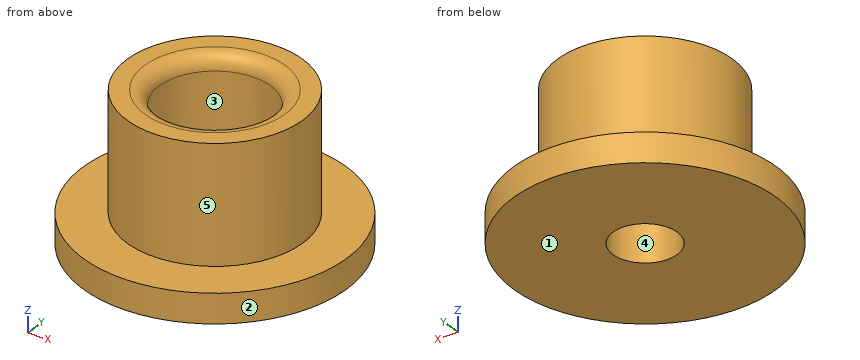
```python
from build123d import *

# Parameters (mm, degrees)
F0_R     = 9
F0_R_2   = 6
F1_DEPTH = 2
F0_R_3   = 3.8
F2_DEPTH = 10
F0_R_4   = 2.2
F3_DEPTH = 5
F4_R     = 1
F5_R     = 1


with BuildPart() as f1:
    # F0 (on Top) → F1 (new body)
    with BuildSketch(Plane.XY):
        Circle(F0_R)
        Circle(F0_R_2, mode=Mode.SUBTRACT)
    extrude(amount=F1_DEPTH)

    # F0 (on Top) → F2 (join)
    with BuildSketch(Plane.XY):
        Circle(F0_R_2)
        Circle(F0_R_3, mode=Mode.SUBTRACT)
    extrude(amount=F2_DEPTH)

    # F0 (on Top) → F3 (join)
    with BuildSketch(Plane.XY):
        Circle(F0_R_3)
        Circle(F0_R_4, mode=Mode.SUBTRACT)
    extrude(amount=F3_DEPTH)

    # F4
    f4_edges = [f1.edges().sort_by_distance(p)[0] for p in [
        (-3.8, 0, 10),
    ]]
    fillet(f4_edges, radius=F4_R)

    # F5
    f5_edges = [f1.edges().sort_by_distance(p)[0] for p in [
        (-2.2, 0, 5),
    ]]
    fillet(f5_edges, radius=F5_R)


solid = f1.part
```
Work out the finished part from the listing and answer in its coordinate system (mm). Face numbers are marked on the shaded views. A direction names the side the tool comes from. Give positions to 0.01 mm unless a question says otherwise; leave off trailing zeros. Loops run counter-clockwise (first coordinate to the right, second up) from the corner with the lowest first, then second, coordinate; pieces in that order, holes last. Notation, with made-up numbers: (82.5, 81.25) -> (131.5, 81.25) arc R13 ccw to (131.5, 87.25) -> close; hole circle Ø11 at (54, 69). An arc over 180 degrees is marked (long way). One line per question, with ' | ' between items. Start each with the question number.
1) Determine the mould class of the marked faces 1, 2 and 3 for opening direction Y: +Y half, -Y half, draft (parallel to the pull), parting line (faces both ways), or undercut.
2) Section C-C, the plane z = 6.25 is taken. Determine the outline of the cut face in (x, y), then the cut area to 3 significant figures.
3) Section D-D, the plane z = 3.5 is taken. Determine the outline of the cut face in (x, y).
4) Each of these flat-tipped pins is pushed along its axis until it touches: pin 1 (3 mm diameter, centred on y = -3, z = 4.5, fed in from -X); pin 2 (2 mm diameter, centred on y = 6, z = 6, fed in from -X); pin 3 (5 mm diameter, centred on x = 6.5, z = 5.5, fed in from +Y). Where does it stop, or does it pass through?
5) Section A-A, the plane y = 0 is taken. Determine the outline of the cut face in (x, z).
6) Straight lines are drawn through the part: L1, parallel to Y at x = 0, z = 2.5; L2, parallel to Y at x = 0, z = 6; L3, parallel to Z at x = 5, y = 6.25. For each, find the intervals that lie inside material, in ascending order.
7) For the marked faces 4 and 5, determine the directions among +Z, -Z, +X, -X, +Y, -Y from which every point of the face is accessible in a straight line to the end or side of a thin tool.
Resolved:
1) face 1: draft | face 2: parting line | face 3: undercut
2) outline: circle Ø12 at (0, 0); hole circle Ø7.6 at (0, 0) | area: 67.7 mm2
3) outline: circle Ø12 at (0, 0); hole circle Ø4.4 at (0, 0)
4) pin 1: x = -5.81 | pin 2: x = -3.32 | pin 3: y = 4.47
5) outline: (-9, 0) -> (-2.2, 0) -> (-2.2, 4) arc R1 ccw to (-3.2, 5) -> (-3.8, 5) -> (-3.8, 9) arc R1 ccw to (-4.8, 10) -> (-6, 10) -> (-6, 2) -> (-9, 2) -> close; (2.2, 0) -> (9, 0) -> (9, 2) -> (6, 2) -> (6, 10) -> (4.8, 10) arc R1 ccw to (3.8, 9) -> (3.8, 5) -> (3.2, 5) arc R1 ccw to (2.2, 4) -> close
6) L1: -6 to -2.2, 2.2 to 6 | L2: -6 to -3.8, 3.8 to 6 | L3: 0 to 2
7) face 4: +Z, -Z | face 5: +Z
